```python
from build123d import *

# Parameters (mm, degrees)
F0_R        = 6
F1_DEPTH    = 300
F2_R        = 11
F3_DEPTH    = 10
F4_T4_DEPTH = 11.3923048454
F4_S5_R     = 6
F4_T6_DEPTH = 7
F5_T4_DEPTH = 11.3923048454
F5_S5_R     = 6
F5_T6_DEPTH = 7
F6_R        = 0.2
F9_D        = 4.2


# Not quite as in the source:
# - a fillet or chamfer that OpenCascade refuses, or shapes differently, is made with other operations: its cross-section is extruded or revolved along the edge and cut away or added


with BuildPart() as f1:
    # F0 (on Top) → F1 (new body)
    with BuildSketch(Plane.XY):
        Circle(F0_R)
    extrude(amount=F1_DEPTH)

    # F2 (on face) → F3 (cut)
    with BuildSketch(Plane.XY.offset(300)):
        Circle(F2_R)
        Polygon((5.1961524227, -3), (-5.1961524227, -3), (0, 6), align=None, mode=Mode.SUBTRACT)
    extrude(amount=-F3_DEPTH, mode=Mode.SUBTRACT)

    # F4: fillet of radius 0.2 on 1 edges, made by hand


with BuildPart() as f4_tool2:
    # F4_s3 → F4_t4 (new body)
    with BuildSketch(Plane.YZ.offset(5.6961524227)):
        with BuildLine():
            ThreePointArc((-3.2, 290), (-3.0585786438, 290.0585786438), (-3, 290.2))
            Line((-3, 290.2), (-3, 290))
            Line((-3, 290), (-3.2, 290))
        make_face()
    extrude(amount=-F4_T4_DEPTH)

    # F4_s5 → F4_t6 (intersect, symmetric)
    with BuildSketch(Plane.XY.offset(290.1)):
        Circle(F4_S5_R)
    extrude(amount=F4_T6_DEPTH, both=True, mode=Mode.INTERSECT)

    split(bisect_by=Plane(origin=(2.5980762114, 1.5, 0), x_dir=(0, 0, 1), z_dir=(-0.8660254038, -0.5, 0)), keep=Keep.TOP)

    split(bisect_by=Plane(origin=(-2.5980762114, 1.5, 0), x_dir=(0, 0, 1), z_dir=(0.8660254038, -0.5, 0)), keep=Keep.TOP)


with BuildPart() as f1_1:
    add(f1.part)

    # F4_t1: union F4_tool2
    add(f4_tool2.part)

    # F5: fillet of radius 0.2 on 1 edges, made by hand


with BuildPart() as f5_tool2:
    # F5_s3 → F5_t4 (new body)
    with BuildSketch(Plane(origin=(-2.8480762114, -4.9330127019, 0), x_dir=(0, 0, 1), z_dir=(0.5, 0.8660254038, 0))):
        with BuildLine():
            ThreePointArc((290, -3.2), (290.0585786438, -3.0585786438), (290.2, -3))
            Line((290.2, -3), (290, -3))
            Line((290, -3), (290, -3.2))
        make_face()
    extrude(amount=F5_T4_DEPTH)

    # F5_s5 → F5_t6 (intersect, symmetric)
    with BuildSketch(Plane.XY.offset(290.1)):
        Circle(F5_S5_R)
    extrude(amount=F5_T6_DEPTH, both=True, mode=Mode.INTERSECT)

    split(bisect_by=Plane(origin=(2.5980762114, 1.5, 0), x_dir=(0, 0, 1), z_dir=(-0.8660254038, -0.5, 0)), keep=Keep.TOP)


with BuildPart() as f1_2:
    add(f1_1.part)

    # F5_t1: union F5_tool2
    add(f5_tool2.part)

    # F6
    f6_edges = [f1_2.edges().sort_by_distance(p)[0] for p in [
        (2.598076, 1.5, 290),
    ]]
    fillet(f6_edges, radius=F6_R)

    # F9 (through all)
    with Locations(Plane.XZ.offset(6)):
        with Locations((0, 16.5)):
            Hole(F9_D / 2)


solid = f1_2.part
```
Geometry check sheet. Reference: the model listing, model coordinates, mm. A direction names the side the tool comes from. Round coordinates to 2 decimals unless told otherwise and drop trailing zeros. Loops run counter-clockwise (first coordinate to the right, second up) from the corner with the lowest first, then second, coordinate; pieces in that order, holes last. Notation, with made-up numbers: M -17,-26.5 L 1,-26.5 A26 ccw 1,12.5 Z; hole C 16,75 d3. An arc over 180 degrees is marked long. Return JSON: item names as keys, results as strings. Group by question number.
(1) Section check A-A, the plane z = 72.5. Enter the section's corners in (x, y).
(2) Set-up check for faces 1 (the face through (-4, 3, 290)), 2 (the face through (0, -3, 295)), 3 (the face through (2.562, 1.563, 295.169)), 4 (the face through (-1.301, -5.857, 147.131)): record each of +Z, -Z, +X, -X, +Y, -Y from which the full face is reachable in a straight line by a thin tool's end or side.
(3) Scan lines: line 1 along Z through (x, y) = (0, 3); line 2 along Z through (x, y) = (1, -4); line 3 along X through (y, z) = (0.25, 16.5). Record each from-to range of solid material in increasing order. Write a range as [from, to].
(4) Go/stop test with flat-tipped pins: pin 1 (2 mm diameter, centred on x = -2.5, y = -5, fed in from +Z); pin 2 (1 mm diameter, centred on x = 2, z = 82, fed in from +Y); pin 3 (5 mm diameter, centred on y = 3.5, z = 116.5, fed in from -X). Record where each tip stops, or that it passes through.
Data:
{
 "1": {"outline": "C 0,0 d12"},
 "2": {"face 1": "+Z, -X, +Y", "face 2": "+Z, +X, -X, -Y", "face 3": "+Z, +X, +Y", "face 4": "+Z, -Z"},
 "3": {"line 1": "[0, 14.4], [18.6, 300]", "line 2": "[0, 14.65], [18.35, 290]", "line 3": "[-5.99, -2.1], [2.1, 5.99]"},
 "4": {"pin 1": "z = 290", "pin 2": "y = 5.81", "pin 3": "x = -5.92"}
}
